Source: CAD feature listing. Evaluate the final solid. Frame: model axes, mm. Give positions to 0.01 mm unless a question says otherwise; leave off trailing zeros. Loops run counter-clockwise (first coordinate to the right, second up) from the corner with the lowest first, then second, coordinate; pieces in that order, holes last. Notation, with made-up numbers: M 83.5,30 L 101.5,30 A15 ccw 101.5,46 Z; hole C 8.5,27 d3. An arc over 180 degrees is marked long. Answer in a Markdown table with one row per item.
```python
from build123d import *

# Parameters (mm, degrees)
SKETCH_AS_DRAWN_W              = 40
SKETCH_AS_DRAWN_H              = 40
SKETCH_AS_DRAWN_R              = 1.95
EXTRUDE_DEPTH                  = 5
EXTRUDE_ONTO_SKETCH_ROLL_ANGLE = 90


with BuildPart() as part:
    # Sketch as drawn → Extrude (new)
    with BuildSketch(Plane.XY):
        with Locations((8.934355, -4.827021)):
            Rectangle(SKETCH_AS_DRAWN_W, SKETCH_AS_DRAWN_H)
        with Locations((8.934355, -4.860531)):
            Circle(SKETCH_AS_DRAWN_R, mode=Mode.SUBTRACT)
    extrude(amount=EXTRUDE_DEPTH)


with BuildPart() as part_1:
    # Extrude onto Sketch roll: moved
    add(part.part.rotate(Axis((0, 0, 0), (1, 0, 0)), EXTRUDE_ONTO_SKETCH_ROLL_ANGLE))


with BuildPart() as part_2:
    # Extrude onto Sketch placement: moved
    add(part_1.part)


solid = part_2.part
```
1) Section A-A, the plane x = 7.5. Return loops of the section in (y, z), then the cut area to 3 significant figures.
Reply:
| item | result |
|---|---|
| outline | M -5,-24.83 L 0,-24.83 L 0,-6.18 L -5,-6.18 Z; M -5,-3.54 L 0,-3.54 L 0,15.17 L -5,15.17 Z |
| area | 187 mm² |
2) Pin query (flat end, axial travel): pin 1 Ø5 at (x, z) = (8.93, -4.86) entering from +Y. Return the tip coordinate at first contact, or that it passes through.
Reply:
| item | result |
|---|---|
| pin 1 | stops at y = 0 |
3) Pull-direction query (Z, two-part tool) for faces 1 (the flat face through (-11.066, -2, -5)), 2 (the flat face through (9, -2, 15.173)), 3 (the cylindrical face through (8.512, -2.465, -6.764)); classes: released by +Z, released by -Z, zero draft, split by the parting line, or undercut.
Reply:
| item | result |
|---|---|
| face 1 | zero draft |
| face 2 | released by +Z |
| face 3 | undercut |
